The listing builds one solid part. Answer for the finished solid, in the listing's coordinates (mm). A direction names the side the tool comes from. Round coordinates to 2 decimals unless told otherwise and drop trailing zeros. Loops run counter-clockwise (first coordinate to the right, second up) from the corner with the lowest first, then second, coordinate; pieces in that order, holes last. Notation, with made-up numbers: (-17, 88) -> (10, 88) arc R31 ccw to (10, 122) -> close; hole circle Ø9 at (-7.75, 79). An arc over 180 degrees is marked (long way). One line per question, with ' | ' between items.
from build123d import *

# Parameters (mm, degrees)
F0_R     = 2
F1_DEPTH = 1.5


with BuildPart() as f1:
    # F0 (on Front) → F1 (new body)
    with BuildSketch(Plane.XZ):
        Polygon((0, 53), (0, 0), (66, 0), (66, 2.5), (68.474874, 4.974874), (68.474874, 37.525126), (66, 40), (66, 49.5), (66, 51.5), (64.5, 53), align=None)
        with Locations((14.5, 3)):
            Circle(F0_R, mode=Mode.SUBTRACT)
        with Locations((65.474874, 6.980275)):
            Circle(F0_R, mode=Mode.SUBTRACT)
        with Locations((14.5, 50)):
            Circle(F0_R, mode=Mode.SUBTRACT)
        with Locations((65.474874, 35.50862)):
            Circle(F0_R, mode=Mode.SUBTRACT)
    extrude(amount=F1_DEPTH)


solid = f1.part
Q1. A cutting plane is placed at C-C on y = -1.1. Give the vertices of the cut face in (x, z).
Numbers:
outline: (0, 0) -> (66, 0) -> (66, 2.5) -> (68.47, 4.97) -> (68.47, 37.53) -> (66, 40) -> (66, 51.5) -> (64.5, 53) -> (0, 53) -> close; hole circle Ø4 at (14.5, 3); hole circle Ø4 at (14.5, 50); hole circle Ø4 at (65.47, 6.98); hole circle Ø4 at (65.47, 35.51)
Q2. A cutting plane is placed at D-D on z = 41. Give the vertices of the cut face in (x, y), plus the area to 3 significant figures.
Numbers:
outline: (0, -1.5) -> (66, -1.5) -> (66, 0) -> (0, 0) -> close | area: 99.0 mm^2
Q3. A cutting plane is placed at B-B on z = 50. Give the vertices of the cut face in (x, y).
Numbers:
outline: (0, -1.5) -> (12.5, -1.5) -> (12.5, 0) -> (0, 0) -> close; (16.5, -1.5) -> (66, -1.5) -> (66, 0) -> (16.5, 0) -> close
Q4. For a pull along X with two mould halves and no side action, classify faces 4 (the face through (0, -1, 27)), 5 (the face through (66.398, -0.74, 33.734)), 6 (the face through (34, 0, 27)) as pulls with the +X half, pulls with the -X half, needs draft (parallel to the pull), parting line crosses it, or undercut.
Numbers:
face 4: pulls with the -X half | face 5: undercut | face 6: needs draft
Q5. Find the intervals of material crossed by line 1 (Z direction, x = 14.5, y = -0.95); line 2 (X direction, y = -0.9, z = 42.5); line 3 (X direction, y = -0.5, z = 48.5), in increasing order. Write a range as from..to.
Numbers:
line 1: 0..1, 5..48, 52..53 | line 2: 0..66 | line 3: 0..13.18, 15.82..66
Q6. A cutting plane is placed at A-A on x = 14.5. Give the vertices of the cut face in (y, z), plus the area to 3 significant figures.
Numbers:
outline: (-1.5, 0) -> (0, 0) -> (0, 1) -> (-1.5, 1) -> close; (-1.5, 5) -> (0, 5) -> (0, 48) -> (-1.5, 48) -> close; (-1.5, 52) -> (0, 52) -> (0, 53) -> (-1.5, 53) -> close | area: 67.5 mm^2
Q7. For faces 1 (the face through (68.475, -1, 21)), 2 (the face through (66, -1, 1)), 3 (the face through (66, -1, 46)), determine the directions among +Z, -Z, +X, -X, +Y, -Y from which every point of the face is accessible in a straight line to the end or side of a thin tool.
Numbers:
face 1: +Z, -Z, +X, +Y, -Y | face 2: -Z, +X, +Y, -Y | face 3: +Z, +X, +Y, -Y
